Input: part model. Units: mm. Frame: model coordinates. A direction names the side the tool comes from. Coordinates: 2 decimals unless noted, no trailing zeros. Write each loop counter-clockwise with the first axis right and the second up, starting at its lowest first coordinate (ties: lowest second). Pieces come first, ordered by that corner, then holes. Notation, with made-up numbers: (81.5, -13) - (132.5, -13) arc R13 cw to (132.5, 8) - close; hole circle Ø6 at (67, 27.25). An arc over 180 degrees is marked (long way). One line per question, with ' | ' between items. Start each with the question number.
1) Section query B-B on y = 2. Return loops of the section in (x, z).
2) First-contact query: P1, Ø10, axis at y = 7, z = 1.5, coming from the +X side; P2, Ø9, axis at y = -15.5, z = -1, coming from the +X side; P3, Ø8, axis at y = 0, z = 0, coming from the +X side; P4, Ø5, axis at y = 10, z = -4.5, coming from the +X side. Flat tips, straight axial feed; report the tip coordinate or a pass-through.
3) Section query A-A on z = 1.25. Return loops of the section in (x, y), and give its area (3 significant figures).
4) Draft query along Z for faces 1 (the cylindrical face through (2.991, -4.436, -2.307)), 2 (the flat face through (1, 0, -10)), 3 (the flat face through (1, 0, 10)), 4 (the flat face through (2.5, -13, 0)). Return one class per face: released by +Z, released by -Z, zero draft, split by the parting line, or undercut.
5) Line query: line 1 (Z direction, x = 12.5, y = 0); line 2 (Y direction, x = 18, z = -4.25); line 3 (Z direction, x = -12, y = -2.5). Output: solid intervals per line, ascending.
6) Section query C-C on z = -8. Return loops of the section in (x, y).
7) Section query D-D on x = 3. Return loops of the section in (y, z).
8) Reachability of faces 5 (the flat face through (10, -7.5, 0)), 6 (the flat face through (-10, 0, 7)), 7 (the flat face through (-8.78, 4.79, -2.08)) from +Z, -Z, +X, -X, +Y, -Y: full face, straight path, thin tool, end or side. Return the list, or none.
```python
from build123d import *

# Parameters (mm, degrees)
SKETCH1_R           = 20
BOSS_EXTRUDE1_DEPTH = 10
CUT_EXTRUDE1_DEPTH  = 33
SKETCH5_W           = 27.400462
SKETCH5_H           = 25.39372
CUT_EXTRUDE3_DEPTH  = 66
FILLET1_R           = 9
SKETCH6_W           = 26.303109
SKETCH6_H           = 19.36506
CUT_EXTRUDE4_DEPTH  = 33
CHAMFER1_SIZE       = 1.25
CHAMFER2_SIZE       = 1.25
SKETCH7_R           = 5
CUT_EXTRUDE5_DEPTH  = 33


with BuildPart() as part:
    # Sketch1 → Boss-Extrude1 (new, symmetric)
    with BuildSketch(Plane.XY):
        Circle(SKETCH1_R)
    extrude(amount=BOSS_EXTRUDE1_DEPTH, both=True)

    # Sketch2 → Cut-Extrude1 (cut, symmetric)
    with BuildSketch(Plane.XY.offset(10)):
        Polygon((0, 20), (0, 24.336587), (-29.859429, 24.336587), (-29.859429, -31.718049), align=None)
    extrude(amount=CUT_EXTRUDE1_DEPTH, both=True, mode=Mode.SUBTRACT)

    # Sketch5 → Cut-Extrude3 (cut)
    with BuildSketch(Plane.XY):
        with Locations((-13.700231, 12.69686)):
            Rectangle(SKETCH5_W, SKETCH5_H)
    extrude(amount=CUT_EXTRUDE3_DEPTH, mode=Mode.SUBTRACT)

    # Fillet1
    fillet1_edges = [part.edges().sort_by_distance(p)[0] for p in [
        (0, 0, 5),
    ]]
    fillet(fillet1_edges, radius=FILLET1_R)

    # Sketch6 → Cut-Extrude4 (cut, symmetric)
    with BuildSketch(Plane.XY):
        with Locations((15.651554, -17.18253)):
            Rectangle(SKETCH6_W, SKETCH6_H)
    extrude(amount=CUT_EXTRUDE4_DEPTH, both=True, mode=Mode.SUBTRACT)

    # Chamfer1
    # the kernel refuses this chamfer: 1.441493, 1.25 mm, written as the material it takes off along each edge
    with BuildSketch(Plane(origin=(2.5, -19.843135, -13.564195), x_dir=(0, 1, 0), z_dir=(0, 0, 1))) as chamfer1_piece_1:
        with BuildLine():
            Line((CHAMFER1_SIZE, 0), (-0.125211, 1.375211))
            ThreePointArc((-0.125211, 1.375211), (-0.076474, 0.708578), (0, 0))
            Line((0, 0), (CHAMFER1_SIZE, 0))
        make_face()
    extrude(amount=27.128391, mode=Mode.SUBTRACT)

    # Chamfer2
    # the kernel refuses this chamfer: 2.264391, 1.25 mm, written as the material it takes off along each edge
    with BuildSketch(Plane(origin=(18.540496, -7.5, -15.267547), x_dir=(0.32758486719281943, 0.944821758209591, 0), z_dir=(0, 0, 1))) as chamfer2_piece_1:
        with BuildLine():
            Line((2.025154, 0), (-CHAMFER2_SIZE * 0.327584867193, CHAMFER2_SIZE * 0.94482175821))
            Line((-CHAMFER2_SIZE * 0.327584867193, CHAMFER2_SIZE * 0.94482175821), (0, 0))
            ThreePointArc((0, 0), (1.053336, -0.025608), (2.025154, 0))
        make_face()
    extrude(amount=30.535093, mode=Mode.SUBTRACT)

    # Sketch7 → Cut-Extrude5 (cut, symmetric)
    with BuildSketch(Plane(origin=(0, 0, 0), x_dir=(0, 0, -1), z_dir=(1, 0, 0))):
        Circle(SKETCH7_R)
    extrude(amount=CUT_EXTRUDE5_DEPTH, both=True, mode=Mode.SUBTRACT)


solid = part.part
```
Answer key:
1) outline: (-10.39, -10) - (19.9, -10) - (19.9, -4.58) - (-10.39, -4.58) - close; (-3.34, 4.58) - (19.9, 4.58) - (19.9, 10) - (-3.34, 10) - close
2) P1: x = 19.81 | P2: x = 2.5 | P3: through | P4: x = 18.54
3) outline: (-17.32, -10) arc R20 ccw to (1.12, -19.97) - (2.5, -18.59) - (2.5, -7.5) - (17.29, -7.5) - (19.2, -5.59) arc R20 ccw to (19.41, -4.84) - (-14.34, -4.84) - close; (-1.02, 4.84) - (19.41, 4.84) arc R20 ccw to (0, 20) - (0, 9) arc R9 cw to start | area: 504 mm²
4) face 1: undercut | face 2: released by -Z | face 3: released by +Z | face 4: zero draft
5) line 1: -10 to -5, 5 to 10 | line 2: -6.79 to -2.63, 2.63 to 8.72 | line 3: -10 to -4.33, 4.33 to 10
6) outline: (-17.32, -10) arc R20 ccw to (1.12, -19.97) - (2.5, -18.59) - (2.5, -7.5) - (17.29, -7.5) - (19.2, -5.59) arc R20 ccw to (0, 20) - close
7) outline: (-7.5, -10) - (19.77, -10) - (19.77, 10) - (-7.5, 10) - close; hole circle Ø10 at (0, 0)
8) face 5: +Z, -Z, +X, -Y | face 6: +Z, -X, +Y | face 7: +Z, -Z, -X, +Y
